```python
from build123d import *

# Parameters (mm, degrees)
SKETCH_R     = 10
PAD_DEPTH    = 168
SKETCH001_R  = 15
PAD001_DEPTH = 148
SKETCH002_W  = 40
SKETCH002_H  = 15
POCKET_DEPTH = 130
SKETCH003_R  = 2.5
HOLE_DEPTH   = 25
HOLE_TIPS_R  = 2.5


with BuildPart() as part:
    # Sketch → Pad (new body, symmetric)
    with BuildSketch(Plane.YZ):
        Circle(SKETCH_R)
    extrude(amount=PAD_DEPTH, both=True)

    # Sketch001 → Pad001 (join, symmetric)
    with BuildSketch(Plane.YZ):
        Circle(SKETCH001_R)
    extrude(amount=PAD001_DEPTH, both=True)

    # Sketch002 → Pocket (cut, symmetric)
    with BuildSketch(Plane.YZ):
        with Locations((0, 17.5)):
            Rectangle(SKETCH002_W, SKETCH002_H)
    extrude(amount=POCKET_DEPTH, both=True, mode=Mode.SUBTRACT)

    # Sketch003 → Hole (cut)
    with BuildSketch(Plane.XY.offset(10)):
        Circle(SKETCH003_R)
        with Locations((-50, 0)):
            Circle(SKETCH003_R)
        with Locations((-100, 0)):
            Circle(SKETCH003_R)
        with Locations((50, 0)):
            Circle(SKETCH003_R)
        with Locations((100, 0)):
            Circle(SKETCH003_R)
    extrude(amount=-HOLE_DEPTH, mode=Mode.SUBTRACT)

    # Hole tips → Hole tip 1 section 0
    with BuildSketch(Plane.XY.offset(-15), mode=Mode.PRIVATE) as hole_tip_1_s0:
        Circle(HOLE_TIPS_R)
    loft([hole_tip_1_s0.sketch, Vertex(0, 0, -16.502152)], mode=Mode.SUBTRACT)

    # Hole tips → Hole tip 2 section 0
    with BuildSketch(Plane.XY.offset(-15), mode=Mode.PRIVATE) as hole_tip_2_s0:
        with Locations((-50, 0)):
            Circle(HOLE_TIPS_R)
    loft([hole_tip_2_s0.sketch, Vertex(-50, 0, -16.502152)], mode=Mode.SUBTRACT)

    # Hole tips → Hole tip 3 section 0
    with BuildSketch(Plane.XY.offset(-15), mode=Mode.PRIVATE) as hole_tip_3_s0:
        with Locations((-100, 0)):
            Circle(HOLE_TIPS_R)
    loft([hole_tip_3_s0.sketch, Vertex(-100, 0, -16.502152)], mode=Mode.SUBTRACT)

    # Hole tips → Hole tip 4 section 0
    with BuildSketch(Plane.XY.offset(-15), mode=Mode.PRIVATE) as hole_tip_4_s0:
        with Locations((50, 0)):
            Circle(HOLE_TIPS_R)
    loft([hole_tip_4_s0.sketch, Vertex(50, 0, -16.502152)], mode=Mode.SUBTRACT)

    # Hole tips → Hole tip 5 section 0
    with BuildSketch(Plane.XY.offset(-15), mode=Mode.PRIVATE) as hole_tip_5_s0:
        with Locations((100, 0)):
            Circle(HOLE_TIPS_R)
    loft([hole_tip_5_s0.sketch, Vertex(100, 0, -16.502152)], mode=Mode.SUBTRACT)


solid = part.part
```
Design review of the part built by this model. Coordinates are the model's own, in mm. A direction names the side the tool comes from. Give positions to 0.01 mm unless a question says otherwise; leave off trailing zeros. Write each loop counter-clockwise with the first axis right and the second up, starting at its lowest first coordinate (ties: lowest second). Pieces come first, ordered by that corner, then holes. Notation, with made-up numbers: (-25.5, 37.5) -> (-1.5, 37.5) arc R24 ccw to (-1.5, 47.5) -> close; hole circle Ø9 at (-17.5, 70). An arc over 180 degrees is marked (long way). Answer in a Markdown table with one row per item.
(1) Consider section A-A (z = 0). State the section outline as (x, y) points, then the cut area to 3 significant figures.
Results:
| item | result |
|---|---|
| outline | (-168, -10) -> (-148, -10) -> (-148, -15) -> (148, -15) -> (148, -10) -> (168, -10) -> (168, 10) -> (148, 10) -> (148, 15) -> (-148, 15) -> (-148, 10) -> (-168, 10) -> close; hole circle Ø5 at (-100, 0); hole circle Ø5 at (-50, 0); hole circle Ø5 at (0, 0); hole circle Ø5 at (50, 0); hole circle Ø5 at (100, 0) |
| area | 9,580 mm2 |
(2) Mouldability with a two-part tool opening along X and no side actions: class faces 1 (the cylindrical face through (-157.86, -2.17, -9.76)), 2 (the flat face through (2, 2, 10)), 3 (the flat face through (-168, 0, 0)), 4 (the flat face through (168, 0, 0)) as +X half, -X half, draft (parallel to the pull), parting line (faces both ways), or undercut.
Results:
| item | result |
|---|---|
| face 1 | draft |
| face 2 | undercut |
| face 3 | -X half |
| face 4 | +X half |
(3) Consider section B-B (x = -22). State the section outline as (y, z) points, then the cut area to 3 significant figures.
Results:
| item | result |
|---|---|
| outline | (-11.18, 10) arc R15 ccw (long way) to (11.18, 10) -> close |
| area | 629 mm2 |
(4) For faces 5 (the cylindrical face through (2.072, -3.252, -14.643)), 6 (the cylindrical face through (158.14, -2.17, -9.76)), 7 (the flat face through (-148, 3, -10)), list the 3-axis set-ups (+Z, -Z, +X, -X, +Y, -Y) from which the entire face can be reached by the end or side of a thin tool; tool diameter is ignored.
Results:
| item | result |
|---|---|
| face 5 | +X, -X |
| face 6 | +X |
| face 7 | -X |
(5) Consider section C-C (y = 6). State the section outline as (x, z) points, then the cut area to 3 significant figures.
Results:
| item | result |
|---|---|
| outline | (-168, -8) -> (-148, -8) -> (-148, -13.75) -> (148, -13.75) -> (148, -8) -> (168, -8) -> (168, 8) -> (148, 8) -> (148, 13.75) -> (130, 13.75) -> (130, 10) -> (-130, 10) -> (-130, 13.75) -> (-148, 13.75) -> (-148, 8) -> (-168, 8) -> close |
| area | 7,800 mm2 |
(6) To check wall thickness, follow probe 1 along X at (y, z) = (0, 1.5); probe 2 along Y at (x, z) = (0, 0.5); probe 3 along X at (y, z) = (-1, -0.5). State the ranges of each line that lie inside material, in increasing order.
Results:
| item | result |
|---|---|
| probe 1 | -168 to -102.5, -97.5 to -52.5, -47.5 to -2.5, 2.5 to 47.5, 52.5 to 97.5, 102.5 to 168 |
| probe 2 | -14.99 to -2.5, 2.5 to 14.99 |
| probe 3 | -168 to -102.29, -97.71 to -52.29, -47.71 to -2.29, 2.29 to 47.71, 52.29 to 97.71, 102.29 to 168 |
(7) Clearance check with flat-ended pins moving along their axes: pin 1 (1.5 mm diameter, centred on y = -4.5, z = 13.5, fed in from -X); pin 2 (4 mm diameter, centred on x = -50, y = 0, fed in from -Z); pin 3 (8 mm diameter, centred on x = 10, z = -6, fed in from -Y); pin 4 (5 mm diameter, centred on x = 98, z = 9, fed in from +Y). State where each tip first meets the part, or that it passes through.
Results:
| item | result |
|---|---|
| pin 1 | x = -148 |
| pin 2 | through |
| pin 3 | y = -14.87 |
| pin 4 | y = 13.52 |
